```python
from build123d import *

# Parameters (mm, degrees)
SKETCH1_R           = 30
SKETCH1_R_2         = 2.35
BOSS_EXTRUDE1_DEPTH = 4
SKETCH2_R           = 3.25
CUT_EXTRUDE1_DEPTH  = 4
SKETCH3_R           = 27
SKETCH3_R_2         = 25
BOSS_EXTRUDE2_DEPTH = 150
CHAMFER1_SIZE       = 5
FILLET1_R           = 5


with BuildPart() as part:
    # Sketch1 → Boss-Extrude1 (new body)
    with BuildSketch(Plane(origin=(0, 0, 0), x_dir=(1, 0, 0), z_dir=(0, 1, 0))):
        with Locations(Location((0, 0, 0), (0, 0, 270))):
            Circle(SKETCH1_R)
        with Locations(Location((-15, -0.001003279, 0), (0, 0, 270))):
            Circle(SKETCH1_R_2, mode=Mode.SUBTRACT)
        with Locations(Location((5.832408968, 13.819660113, 0), (0, 0, 270))):
            Circle(SKETCH1_R_2, mode=Mode.SUBTRACT)
        with Locations(Location((10, -11.180339887, 0), (0, 0, 270))):
            Circle(SKETCH1_R_2, mode=Mode.SUBTRACT)
    extrude(amount=BOSS_EXTRUDE1_DEPTH)

    # Sketch2 → Cut-Extrude1 (cut)
    with BuildSketch(Plane(origin=(0, 4, 0), x_dir=(1, 0, 0), z_dir=(0, 1, 0))):
        with Locations(Location((0, 0, 0), (0, 0, 270))):
            Circle(SKETCH2_R)
    extrude(amount=-CUT_EXTRUDE1_DEPTH, mode=Mode.SUBTRACT)

    # Sketch3 → Boss-Extrude2 (add)
    with BuildSketch(Plane.XZ):
        with Locations(Location((0, 0, 0), (0, 0, 90))):
            Circle(SKETCH3_R)
        with Locations(Location((0, 0, 0), (0, 0, 270))):
            Circle(SKETCH3_R_2, mode=Mode.SUBTRACT)
    extrude(amount=BOSS_EXTRUDE2_DEPTH)

    # Chamfer1
    # the kernel refuses this chamfer: 5 mm, written as the material it takes off along each edge
    with BuildSketch(Plane(origin=(0, -150, 0), x_dir=(0, 0, 1), z_dir=(1, 0, 0))) as chamfer1_piece_1:
        Polygon((27, -CHAMFER1_SIZE), (27 - CHAMFER1_SIZE, 0), (27, 0), align=None)
    revolve(axis=Axis((0, -150, 0), (0, -1, 0)), mode=Mode.SUBTRACT)

    # Fillet1
    # the kernel refuses this fillet: 5 mm, written as the material it adds along each edge
    with BuildSketch(Plane(origin=(0, 0, 0), x_dir=(0, 0, 1), z_dir=(1, 0, 0))) as fillet1_piece_1:
        with BuildLine():
            CenterArc((32, 4.582575695), FILLET1_R, 180, 66.421821522)
            Line((27, 4.582575695), (26.9, 4.582575695))
            Line((26.9, 4.582575695), (26.9, 0))
            Line((26.9, 0), (27, -0.1))
            ThreePointArc((27, -0.1), (28.5, -0.1), (29.96, -0.091651514))
            Line((29.96, -0.091651514), (30, 0))
        make_face()
    revolve(axis=Axis((0, 0, 0), (0, -1, 0)))


solid = part.part
```
Can you work these out from the model? Positions are in its coordinate system, mm. A direction names the side the tool comes from. Give positions to 0.01 mm unless a question says otherwise; leave off trailing zeros. Write each loop counter-clockwise with the first axis right and the second up, starting at its lowest first coordinate (ties: lowest second). Pieces come first, ordered by that corner, then holes. Notation, with made-up numbers: (33.25, 65.25) -> (38.25, 65.25) arc R10 cw to (38.25, 69.25) -> close; hole circle Ø8 at (-28.75, -34). An arc over 180 degrees is marked (long way). Write item = value, one per line.
(1) Suppose I cut it at A-A on z = 0. Write out the boundary of the cut face in (x, y).
Worked out:
outline = (-30, 0) arc R5 cw to (-27, -4.58) -> (-27, -145) -> (-25, -147) -> (-25, 0) -> (-17.35, 0) -> (-17.35, 4) -> (-30, 4) -> close; (-12.65, 0) -> (-3.25, 0) -> (-3.25, 4) -> (-12.65, 4) -> close; (3.25, 0) -> (25, 0) -> (25, -147) -> (27, -145) -> (27, -4.58) arc R5 cw to (30, 0) -> (30, 4) -> (3.25, 4) -> close
(2) I need wall thicknesses on probe 1 along X at (y, z) = (1, 0); probe 2 along X at (y, z) = (-50, 0); probe 3 along Y at (x, z) = (14.5, -20). Which ranges of each line are inside material? Lowest first, please. Write a range as from..to.
Worked out:
probe_1 = -30..-17.35, -12.65..-3.25, 3.25..30
probe_2 = -27..-25, 25..27
probe_3 = 0..4
(3) Thinking about a two-plate mould opening in X: for faces 3 (the face through (26.36, -73.81, -5.85)), 4 (the face through (-1.978, 2.028, -2.579)), 5 (the face through (0, 4, 6)), which applies, released by +X, released by -X, zero draft, split by the parting line, or undercut?
Worked out:
face_3 = split by the parting line
face_4 = undercut
face_5 = zero draft
(4) Suppose I cut it at C-C on y = -43. Write out the boundary of the cut face in (x, z).
Worked out:
outline = circle Ø54 at (0, 0); hole circle Ø50 at (0, 0)
(5) I'm going to push flat-ended pins straight in: P1, Ø3, axis at x = -4, y = -34.5, coming from the +Z side; P2, Ø8, axis at x = 11.5, y = -102, coming from the -Z side; P3, Ø2, axis at y = -119.5, z = -17, coming from the +X side. Where does each tip first touch, or does it pass through?
Worked out:
P1 = 26.88
P2 = -25.94
P3 = 21.75
(6) For faces 1 (the face through (-5, 0, 0)), 2 (the face through (7.915, 1.972, 12.265)), which set-ups out of +Z, -Z, +X, -X, +Y, -Y let a thin tool reach every point of the face, with its end or its side?
Worked out:
face_1 = -Y
face_2 = +Y, -Y
(7) Suppose I cut it at B-B on x = 0. Write out the boundary of the cut face in (y, z), then the cut area to 3 significant figures.
Worked out:
outline = (-147, -25) -> (-145, -27) -> (-4.58, -27) arc R5 cw to (0, -30) -> (4, -30) -> (4, -3.25) -> (0, -3.25) -> (0, -25) -> close; (-147, 25) -> (0, 25) -> (0, 3.25) -> (4, 3.25) -> (4, 30) -> (0, 30) arc R5 cw to (-4.58, 27) -> (-145, 27) -> close
area = 806 mm^2
